```python
from build123d import *

# Parameters (mm, degrees)
SKETCH1_R                = 47
SKETCH1_R_2              = 38
SKETCH1_R_3              = 2.15
BOSS_EXTRUDE1_DEPTH      = 11.5
CUT_EXTRUDE1_DEPTH       = 10
FILLET1_R                = 1
CIRPATTERN1_COUNT        = 4
CIRPATTERN1_ANGLE        = 270
FILLET1_OF_CIRPATTERN1_R = 1


with BuildPart() as part:
    # Sketch1 → Boss-Extrude1 (new, symmetric)
    with BuildSketch(Plane(origin=(0, 0, 0), x_dir=(1, 0, 0), z_dir=(0, 1, 0))):
        with Locations(Location((0, 0, 0), (0, 0, 270))):
            Circle(SKETCH1_R)
        with Locations(Location((0, 0, 0), (0, 0, 270))):
            Circle(SKETCH1_R_2, mode=Mode.SUBTRACT)
        with Locations(Location((0, 42, 0), (0, 0, 270))):
            Circle(SKETCH1_R_3, mode=Mode.SUBTRACT)
        with Locations(Location((29.69848481, 29.69848481, 0), (0, 0, 270))):
            Circle(SKETCH1_R_3, mode=Mode.SUBTRACT)
        with Locations(Location((42, 0, 0), (0, 0, 270))):
            Circle(SKETCH1_R_3, mode=Mode.SUBTRACT)
        with Locations(Location((29.69848481, -29.69848481, 0), (0, 0, 270))):
            Circle(SKETCH1_R_3, mode=Mode.SUBTRACT)
        with Locations(Location((0, -42, 0), (0, 0, 270))):
            Circle(SKETCH1_R_3, mode=Mode.SUBTRACT)
        with Locations(Location((-29.69848481, -29.69848481, 0), (0, 0, 270))):
            Circle(SKETCH1_R_3, mode=Mode.SUBTRACT)
        with Locations(Location((-42, 0, 0), (0, 0, 270))):
            Circle(SKETCH1_R_3, mode=Mode.SUBTRACT)
        with Locations(Location((-29.69848481, 29.69848481, 0), (0, 0, 270))):
            Circle(SKETCH1_R_3, mode=Mode.SUBTRACT)
    extrude(amount=BOSS_EXTRUDE1_DEPTH, both=True)

    # Sketch2 → Cut-Extrude1 (cut)
    with BuildSketch(Plane(origin=(0, 11.5, 0), x_dir=(1, 0, 0), z_dir=(0, 1, 0))):
        with BuildLine():
            Line((-6.134731034, 46.597908485), (-4.959995304, 37.674904732))
            ThreePointArc((-4.959995304, 37.674904732), (0, 38), (4.959995304, 37.674904732))
            Line((4.959995304, 37.674904732), (6.134731034, 46.597908485))
            ThreePointArc((6.134731034, 46.597908485), (0, 47), (-6.134731034, 46.597908485))
        make_face()
    cut_extrude1 = extrude(amount=-CUT_EXTRUDE1_DEPTH, mode=Mode.SUBTRACT)

    # Fillet1
    fillet1_edges = [part.edges().sort_by_distance(p)[0] for p in [
        (-6.134731034, 6.5, -46.597908485),
        (6.134731034, 6.5, -46.597908485),
        (4.959995304, 6.5, -37.674904732),
        (-4.959995304, 6.5, -37.674904732),
    ]]
    fillet(fillet1_edges, radius=FILLET1_R)

    # CirPattern1: Cut-Extrude1 ×4 about axis
    cirpattern1_axis = Axis((0, 0, 0), (0, 1, 0))
    for i in range(1, CIRPATTERN1_COUNT):
        add(cut_extrude1.rotate(cirpattern1_axis, i * CIRPATTERN1_ANGLE / (CIRPATTERN1_COUNT - 1)), mode=Mode.SUBTRACT)

    # Fillet1 of CirPattern1
    fillet1_of_cirpattern1_edges = [part.edges().sort_by_distance(p)[0] for p in [
        (-46.597908485, 6.5, 6.134731034),
        (-46.597908485, 6.5, -6.134731034),
        (-37.674904732, 6.5, -4.959995304),
        (-37.674904732, 6.5, 4.959995304),
        (6.134731034, 6.5, 46.597908485),
        (-6.134731034, 6.5, 46.597908485),
        (-4.959995304, 6.5, 37.674904732),
        (4.959995304, 6.5, 37.674904732),
        (46.597908485, 6.5, -6.134731034),
        (46.597908485, 6.5, 6.134731034),
        (37.674904732, 6.5, 4.959995304),
        (37.674904732, 6.5, -4.959995304),
    ]]
    fillet(fillet1_of_cirpattern1_edges, radius=FILLET1_OF_CIRPATTERN1_R)


solid = part.part
```
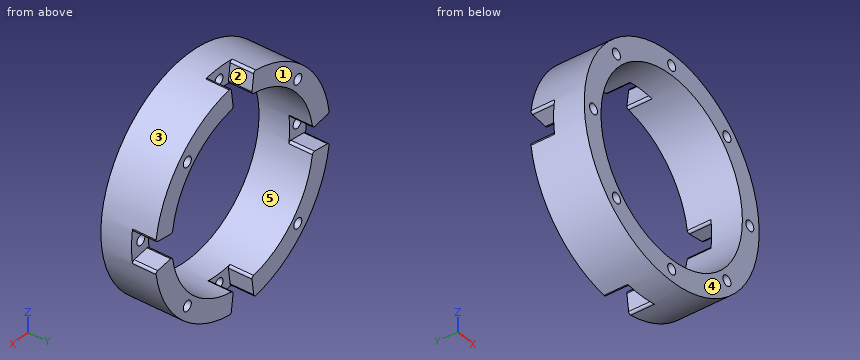
Input: part model. Units: mm. Frame: model coordinates. Face numbers are marked on the shaded views. A direction names the side the tool comes from. Round coordinates to 2 decimals unless told otherwise and drop trailing zeros. Loops run counter-clockwise (first coordinate to the right, second up) from the corner with the lowest first, then second, coordinate; pieces in that order, holes last. Notation, with made-up numbers: (45, -31) -> (87, -31) arc R35 cw to (87, 3) -> close; hole circle Ø5 at (-16.75, 40). An arc over 180 degrees is marked (long way). Use one line per item in the form item = value. Start each with the question number.
Item 1: Section query B-B on x = -23. Return the cut outline in (y, z), then the cut area to 3 significant figures.
Item 2: Section query D-D on y = -8.5. Count the separate pieces of the cut face and the enclosed holes in it, then the cut area to 3 significant figures.
Item 3: Section query C-C on x = 0. Return the cut outline in (y, z), then the cut area to 3 significant figures.
Item 4: Contact query for flat-ended pins moving along their axis: pin 1 Ø3.5 at (x, z) = (42, 0) entering from -Y; pin 2 Ø10 at (x, y) = (26, -0.5) entering from +Z; pin 3 Ø7 at (x, z) = (-42, 0) entering from -Y; pin 4 Ø1.5 at (x, y) = (-33, -2) entering from -Z. Output: stop coordinate, or through.
Item 5: Set-up query: the marked faces 1 and 2. Return all of +Z, -Z, +X, -X, +Y, -Y with unobstructed straight access to the full face (end or side cutting, diameter ignored); none if empty.
Item 6: Section query A-A on z = -18.5. Return the cut outline in (x, y).
Item 7: Material intervals for L1, parallel to X at y = -7.75, z = 0; L2, parallel to Z at x = -28.5, y = 8.5; L3, parallel to Z at x = 31.5, y = 3.5, sorted ascending. Write a range as from..to.
Item 8: Mould query, pull axis X, two halves, no side actions, for the marked faces 3, 4 and 5. Classes: pulls with the +X half, pulls with the -X half, needs draft (parallel to the pull), parting line crosses it, or undercut.
Ans:
q1.outline = (-11.5, -40.99) -> (11.5, -40.99) -> (11.5, -30.25) -> (-11.5, -30.25) -> close; (-11.5, 30.25) -> (11.5, 30.25) -> (11.5, 40.99) -> (-11.5, 40.99) -> close
q1.area = 494 mm^2
q2.separate_pieces = 1
q2.enclosed_holes = 9
q2.area = 2,290 mm^2
q3.outline = (-11.5, -47) -> (1.5, -47) -> (1.5, -44.15) -> (-11.5, -44.15) -> close; (-11.5, -39.85) -> (1.5, -39.85) -> (1.5, -38) -> (-11.5, -38) -> close; (-11.5, 38) -> (1.5, 38) -> (1.5, 39.85) -> (-11.5, 39.85) -> close; (-11.5, 44.15) -> (1.5, 44.15) -> (1.5, 47) -> (-11.5, 47) -> close
q3.area = 122 mm^2
q4.pin_1 = through
q4.pin_2 = 42.05
q4.pin_3 = -11.5
q4.pin_4 = -34.19
q5.face_1 = +Z, -Z, +X, -X, +Y
q5.face_2 = +Z, +Y
q6.outline = (-43.21, -11.5) -> (-33.19, -11.5) -> (-33.19, 11.5) -> (-43.21, 11.5) -> close; (33.19, -11.5) -> (43.21, -11.5) -> (43.21, 11.5) -> (33.19, 11.5) -> close
q7.L1 = -47..-44.15, -39.85..-38, 38..39.85, 44.15..47
q7.L2 = -37.37..-31.48, -27.91..-25.13, 25.13..27.91, 31.48..37.37
q7.L3 = -34.88..-30.87, -28.53..-21.25, 21.25..28.53, 30.87..34.88
q8.face_3 = parting line crosses it
q8.face_4 = needs draft
q8.face_5 = undercut
